Source: three-view drawing plus pictorial views. Frame: mm from the lowest corner of the part. A direction names the side the tool comes from. Give positions to 0.01 mm unless a question says otherwise; leave off trailing zeros. Order: outer loops, then holes, each group sorted by start corner. A loop starts at its lowest first (then second) coordinate and runs counter-clockwise, first axis right, second up. Notation, with made-up numbers: (6.5, -2) -> (53.5, -2) arc R8 cw to (53.5, 4) -> close; hole circle Ø9 at (-20, 12). An arc over 180 degrees is marked (long way). Answer in a Markdown table with one row per item. Add a question column.
Q1. Line query: line 1 along X through (y, z) = (8.5, 26.35); line 2 along Z through (x, y) = (45, 6.5); line 3 along Y through (x, z) = (47, 29.9). Output: solid intervals per line, ascending. Write a range as from..to.
Q2. Cut plane C-C on x = 9. Count the separate pieces of the cut face and the enclosed holes in it, and give its area (3 significant figures).
Q3. Contact query for flat-ended pins moving along their axis: P1, Ø0.5, axis at y = 8.5, z = 29.5, coming from the +X side; P2, Ø5.5, axis at y = 9, z = 28.5, coming from the -X side; P3, Ø2, axis at x = 9.5, y = 9, coming from the +Z side; P4, Ø3, axis at x = 21, y = 7, coming from the +Z side. Output: stop coordinate, or through.
Q4. Cut plane B-B on x = 28. Return the cut outline in (y, z).
Q5. Cut plane A-A on z = 28. Return the cut outline in (x, y), and give its area (3 significant figures).
Q6. Set-up query: the marked faces 1, 2, 3, 4 and 5. Return all of +Z, -Z, +X, -X, +Y, -Y with unobstructed straight access to the full face (end or side cutting, diameter ignored); none if empty.
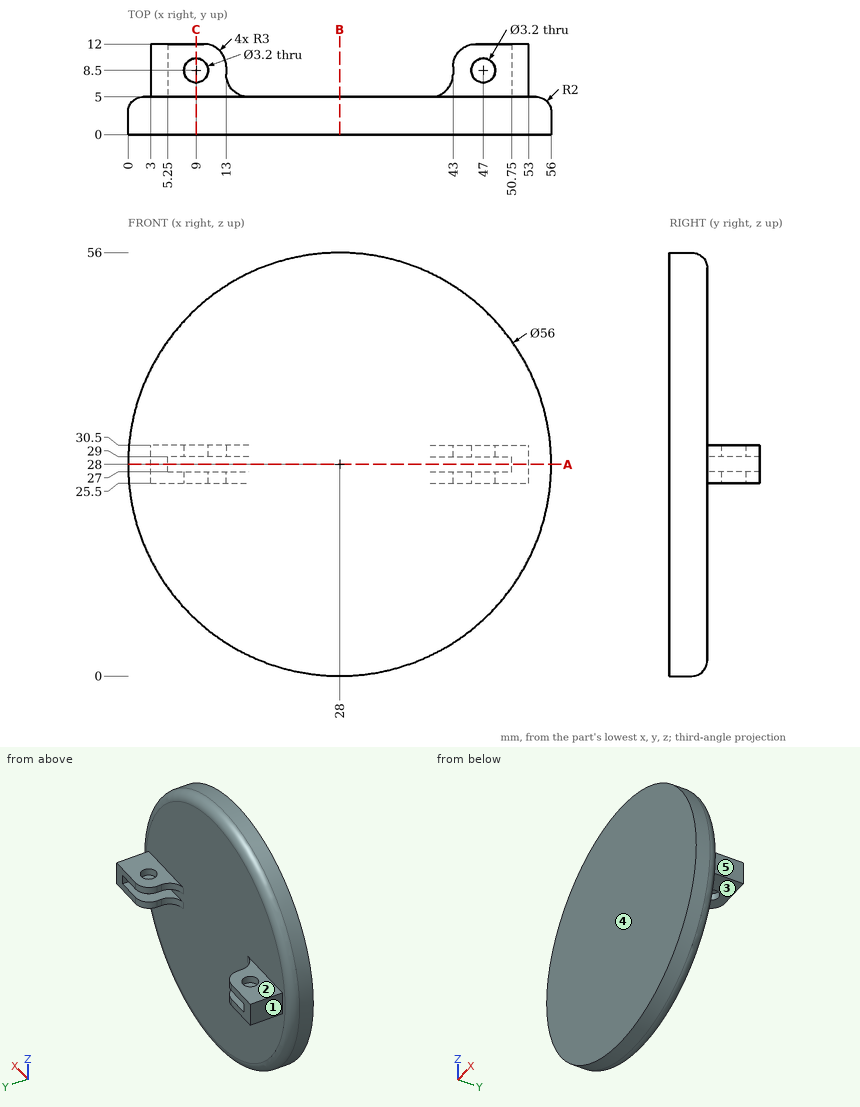
Completed:
| question | item | result |
|---|---|---|
| 1 | line 1 | x = 3..7.4, 10.6..13, 43..45.4, 48.6..53 |
| 1 | line 2 | z = 25.5..27, 29..30.5 |
| 1 | line 3 | y = 0..6.9, 10.1..12 |
| 2 | separate pieces | 3 |
| 2 | enclosed holes | 0 |
| 2 | area | 215 mm² |
| 3 | P1 | stops at x = 53 |
| 3 | P2 | stops at x = 3 |
| 3 | P3 | stops at z = 30.5 |
| 3 | P4 | passes through |
| 4 | outline | (0, 0) -> (3, 0) arc R2 ccw to (5, 2) -> (5, 54) arc R2 ccw to (3, 56) -> (0, 56) -> close |
| 5 | outline | (0, 0) -> (56, 0) -> (56, 3) arc R2 ccw to (54, 5) -> (53, 5) -> (53, 12) -> (50.75, 12) -> (50.75, 5) -> (5.25, 5) -> (5.25, 12) -> (3, 12) -> (3, 5) -> (2, 5) arc R2 ccw to (0, 3) -> close |
| 5 | area | 310 mm² |
| 6 | face 1 | +Z, -Z, -X, +Y |
| 6 | face 2 | +Z, +X, -X, +Y |
| 6 | face 3 | -Z, +X, -X, +Y |
| 6 | face 4 | +Z, -Z, +X, -X, -Y |
| 6 | face 5 | +Z, -Z, +X, +Y |
